Read the model definition and answer for the solid it produces. Units are mm, in the model's axes. Round coordinates to 2 decimals unless told otherwise and drop trailing zeros. Loops run counter-clockwise (first coordinate to the right, second up) from the corner with the lowest first, then second, coordinate; pieces in that order, holes last. Notation, with made-up numbers: M 70,39 L 80,39 A14 ccw 80,49 Z; hole C 84,16.25 d7. An arc over 180 degrees is marked long. Write each question's results on one line, items separated by ' | '.
Autodesk Inventor part; units mm, degrees
ref_plane "YZ Plane" through (0, 0, 0) normal (1, 0, 0) x (0, 1, 0)
ref_plane "XZ Plane" through (0, 0, 0) normal (0, 1, 0) x (-1, 0, 0)
ref_plane "XY Plane" through (0, 0, 0) normal (0, 0, 1) x (1, 0, 0)
sketch "Sketch1" plane through (0, 0, 0) normal (0, 0, 1) x (1, 0, 0)
  line L0 (-89, 89) -> (89, 89)
  line L1 (89, 89) -> (89, -89)
  line L2 (89, -89) -> (-89, -89)
  line L3 (-89, -89) -> (-89, 89)
  line L4 (-56.125, 56.125) -> (-78.5, 56.125)
  line L5 (-78.5, -56.125) -> (-56.125, -56.125)
  line L6 (56.125, 56.125) -> (56.125, 78.5)
  line L7 (-56.125, 78.5) -> (-56.125, 56.125)
  line L8 (56.125, 56.125) -> (78.5, 56.125)
  line L9 (78.5, -56.125) -> (56.125, -56.125)
  line L10 (56.125, -56.125) -> (56.125, -78.5)
  line L11 (-56.125, -78.5) -> (-56.125, -56.125)
  line L12 (-78.5, 36.125) -> (-59, 36.125)
  line L13 (-59, 36.125) -> (-59, -36.125)
  line L14 (-59, -36.125) -> (-78.5, -36.125)
  line L15 (-78.5, 56.125) -> (-78.5, 36.125)
  line L16 (-78.5, -36.125) -> (-78.5, -56.125)
  line L17 (78.5, 36.125) -> (59, 36.125)
  line L18 (59, 36.125) -> (59, -36.125)
  line L19 (59, -36.125) -> (78.5, -36.125)
  line L20 (78.5, 56.125) -> (78.5, 36.125)
  line L21 (78.5, -36.125) -> (78.5, -56.125)
  line L22 (36.125, 78.5) -> (36.125, 59)
  line L23 (36.125, 59) -> (-36.125, 59)
  line L24 (-36.125, 59) -> (-36.125, 78.5)
  line L25 (36.125, -78.5) -> (36.125, -59)
  line L26 (36.125, -59) -> (-36.125, -59)
  line L27 (-36.125, -59) -> (-36.125, -78.5)
  line L28 (56.125, 78.5) -> (36.125, 78.5)
  line L29 (-36.125, 78.5) -> (-56.125, 78.5)
  line L30 (56.125, -78.5) -> (36.125, -78.5)
  line L31 (-36.125, -78.5) -> (-56.125, -78.5)
  point P0 (0, 0)
  point P1 (-78.5, 0)
  dimension "d4" = 112.25
  dimension "d5" = 112.25
  dimension "d29" = 0
  dimension "d30" = 0
  dimension "d33" = 178
  dimension "d34" = 89
  dimension "d35" = 89
  dimension "d41" = 20
  dimension "d42" = 20
  dimension "d43" = 30
  dimension "d46" = 20
  dimension "d47" = 20
  dimension "d48" = 30
  dimension "d49" = 157
  dimension "d50" = 78.5
  dimension "d51" = 30
  dimension "d52" = 30
  dimension "d53" = 20
  dimension "d54" = 157
  dimension "d55" = 78.5
  dimension "d56" = 20
extrude "Extrusion1" add sketch "Sketch1" along normal blind 5
sketch "Sketch2" plane through (0, 0, 5) normal (0, 0, 1) x (1, 0, 0)
  circle A0 centre (-81.5, 0) radius 2
  circle A1 centre (81.5, 0) radius 2
  line L0 (-78.5, 36.125) -> (-78.5, 56.125)
  line L1 (78.5, 56.125) -> (78.5, 36.125)
  circle A2 centre (0, 81.5) radius 2
  circle A3 centre (0, -81.5) radius 2
  line L2 (36.125, 78.5) -> (56.125, 78.5)
  line L3 (56.125, -78.5) -> (36.125, -78.5)
  line L4 (-89, 89) -> (-89, -89)
  line L5 (89, 89) -> (-89, 89)
  line L6 (89, -89) -> (89, 89)
  line L7 (-89, -89) -> (89, -89)
  point P0 (0, 0)
  point P1 (-78.5, -56.125)
  point P2 (78.5, -56.125)
  point P3 (-56.125, 78.5)
  point P4 (-56.125, -78.5)
  dimension "d18" = 4
  dimension "d37" = 7.5
  dimension "d38" = 7.5
  dimension "d39" = 7.5
  dimension "d40" = 7.5
hole "Hole1" at (-81.5, 0, 5) at (0, 81.5, 5) at (81.5, 0, 5) at (0, -81.5, 5) direction (0, 0, -1) diameter 4 end through all
fillet "Fillet1" radius 2 4 edges at (-89, -89, 2.5) (-89, 89, 2.5) (89, -89, 2.5) (89, 89, 2.5)
sketch "Sketch3" plane through (0, 0, 5) normal (0, 0, 1) x (1, 0, 0)
  line L0 (68.475, -68.475) -> (-68.475, -68.475)
  line L1 (-68.475, -68.475) -> (-68.475, 68.475)
  line L2 (-68.475, 68.475) -> (68.475, 68.475)
  line L3 (68.475, 68.475) -> (68.475, -68.475)
  line L4 (68.475, -68.475) -> (-68.475, 68.475) construction
  line L5 (-68.475, -68.475) -> (68.475, 68.475) construction
  circle A0 centre (-68.475, 68.475) radius 4.875
  point P0 (0, 0)
  dimension "d31" = 136.95
  dimension "d32" = 9.75
fillet "Fillet2" radius 10 4 edges at (-56.125, 56.125, 2.5) (56.125, 56.125, 2.5) (56.125, -56.125, 2.5) (-56.125, -56.125, 2.5)
fillet "Fillet3" radius 5 8 edges at (-59, 36.125, 2.5) (-59, -36.125, 2.5) (-36.125, -59, 2.5) (36.125, -59, 2.5) (59, -36.125, 2.5) (59, 36.125, 2.5) (36.125, 59, 2.5) (-36.125, 59, 2.5)
hole "Hole2" at (-68.475, 68.475, 5) at (68.475, 68.475, 5) at (68.475, -68.475, 5) at (-68.475, -68.475, 5) direction (0, 0, -1) diameter 6 end through all
equation "\"d38\" = d37"
equation "\"d39\" = d37"
equation "\"d40\" = d37"
equation "\"d21\" = d18"
equation "\"d6\" = 0.5 * d3"
equation "\"d7\" = 0.5 * d2"
properties part number "WaagePlexiOben1" material "PET Plastic"
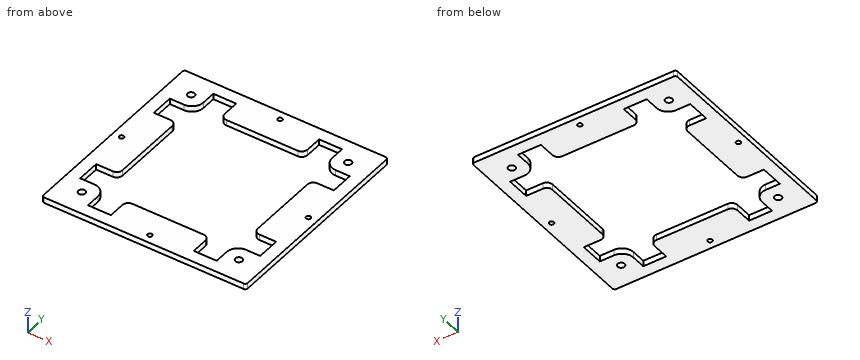
1. Find the intervals of material crossed by L1, parallel to X at y = 68, z = 2.2 (3 decimals); L2, parallel to X at y = 0, z = 2.2; L3, parallel to X at y = 81.5, z = 3.85, in increasing order.
Completed:
L1: x = -89 to -71.437, -65.513 to -56.125, -36.125 to 36.125, 56.125 to 65.513, 71.437 to 89 | L2: x = -89 to -83.5, -79.5 to -59, 59 to 79.5, 83.5 to 89 | L3: x = -89 to -2, 2 to 89
2. Find section A-A, the plane y = -48. Give the vertices of the cut face in (x, z).
Completed:
outline: M -89,0 L -78.5,0 L -78.5,5 L -89,5 Z; M 78.5,0 L 89,0 L 89,5 L 78.5,5 Z
3. Find section B-B, the plane x = -24. Give the vertices of the cut face in (y, z).
Completed:
outline: M -89,0 L -59,0 L -59,5 L -89,5 Z; M 59,0 L 89,0 L 89,5 L 59,5 Z
4. Find section D-D, the plane z = 2.05. Count the separate pieces of the cut face and the enclosed holes in it, then the cut area to 3 significant figures.
Completed:
separate pieces: 1 | enclosed holes: 9 | area: 14,400 mm2
5. Find section C-C, the plane x = 75.5. Give the vertices of the cut face in (y, z) (3 decimals).
Completed:
outline: M -89,0 L -56.125,0 L -56.125,5 L -89,5 Z; M -36.125,0 L 36.125,0 L 36.125,5 L -36.125,5 Z; M 56.125,0 L 89,0 L 89,5 L 56.125,5 Z
